Build history of the part. All positions in model axes, mm. A direction names the side the tool comes from. Give positions to 0.01 mm unless a question says otherwise; leave off trailing zeros. Loops run counter-clockwise (first coordinate to the right, second up) from the corner with the lowest first, then second, coordinate; pieces in that order, holes last. Notation, with made-up numbers: (66.25, 83) -> (73.25, 83) arc R11 ccw to (73.25, 97) -> close; hole circle Ø7 at (19, 59.25). An arc over 180 degrees is marked (long way). Answer as a JSON object with one key per item and string values. Group by question number.
Q1. Drop flat-ended pins along their axis: pin 1 (3 mm diameter, centred on x = 94, y = 0, fed in from +Z); pin 2 (12 mm diameter, centred on x = 1.5, y = 0, fed in from +Z). Give the stop position or say it passes through.
Q2. Two-plate mould, pull along Y, no slides. Class faces 3 (the flat face through (-100, 0, 3)), 4 (the flat face through (-1, 16, 13)), 5 (the flat face through (-1, -17.5, 9)), 6 (the flat face through (-1, 0, 5)): pulls with the +Y half, pulls with the -Y half, needs draft (parallel to the pull), parting line crosses it, or undercut.
Q3. Wall check: probe 1 along Y at (x, z) = (-2.5, 13.5); probe 2 along Y at (x, z) = (94, 3.45); probe 3 along Z at (x, y) = (32, 0.5). Give the ranges that are in metal, low to high. Write a range as from..to.
Q4. Band-saw the part on B-B, the plane z = 9. Write the cut outline in (x, y).
Q5. Tool access for faces 1 (the cylindrical face through (-96.5, 0.1, 2.5)), 2 (the flat face through (-1, 7, 13)): list every direction of +Z, -Z, +X, -X, +Y, -Y with a clear straight run to the whole face (end or side of a thin tool).
Q6. Band-saw the part on A-A, the plane y = 0. Write the cut outline in (x, z), plus the area to 3 significant figures.
from build123d import *

# Parameters (mm, degrees)
F0_W     = 200
F0_H     = 35
F1_DEPTH = 20
F2_R     = 2.5
F3_DEPTH = 25
F4_SIZE  = 1
F6_DEPTH = 240
F8_DEPTH = 250


with BuildPart() as f1:
    # F0 (on Top) → F1 (new body)
    with BuildSketch(Plane.XY):
        Rectangle(F0_W, F0_H)
    extrude(amount=F1_DEPTH)

    # F2 (on face) → F3 (cut)
    with BuildSketch(Plane.XY.offset(20)):
        with Locations((-94, 0)):
            Circle(F2_R)
        with Locations((94, 0)):
            Circle(F2_R)
    extrude(amount=-F3_DEPTH, mode=Mode.SUBTRACT)

    # F4
    f4_edges = [f1.edges().sort_by_distance(p)[0] for p in [
        (0, 17.5, 20),
        (100, 0, 20),
        (-100, 0, 20),
        (0, -17.5, 20),
        (-96.5, 0, 20),
        (91.5, 0, 20),
    ]]
    chamfer(f4_edges, length=F4_SIZE)

    # F5 (on face) → F6 (cut)
    with BuildSketch(Plane(origin=(-100, 0, 0), x_dir=(0, -1, 0), z_dir=(-1, 0, 0))):
        with BuildLine():
            Line((-13, 21.054447), (-16, 21.054447))
            Line((-16, 21.054447), (-16, 6.5))
            ThreePointArc((-16, 6.5), (-15.56066, 5.43934), (-14.5, 5))
            ThreePointArc((-14.5, 5), (-13.43934, 5.43934), (-13, 6.5))
            Line((-13, 6.5), (-13, 21.054447))
        make_face()
        with BuildLine():
            Line((-8.5, 21.054447), (-11.5, 21.054447))
            Line((-11.5, 21.054447), (-11.5, 6.5))
            ThreePointArc((-11.5, 6.5), (-11.06066, 5.43934), (-10, 5))
            ThreePointArc((-10, 5), (-8.93934, 5.43934), (-8.5, 6.5))
            Line((-8.5, 6.5), (-8.5, 21.054447))
        make_face()
        with BuildLine():
            Line((-4, 20.95042), (-7, 20.95042))
            Line((-7, 20.95042), (-7, 6.5))
            ThreePointArc((-7, 6.5), (-6.56066, 5.43934), (-5.5, 5))
            ThreePointArc((-5.5, 5), (-4.43934, 5.43934), (-4, 6.5))
            Line((-4, 6.5), (-4, 20.95042))
        make_face()
        with BuildLine():
            Line((11.5, 21.002434), (8.5, 21.002434))
            Line((8.5, 21.002434), (8.5, 6.5))
            ThreePointArc((8.5, 6.5), (8.93934, 5.43934), (10, 5))
            ThreePointArc((10, 5), (11.06066, 5.43934), (11.5, 6.5))
            Line((11.5, 6.5), (11.5, 21.002434))
        make_face()
        with BuildLine():
            Line((16, 21.002434), (13, 21.002434))
            Line((13, 21.002434), (13, 6.5))
            ThreePointArc((13, 6.5), (13.43934, 5.43934), (14.5, 5))
            ThreePointArc((14.5, 5), (15.56066, 5.43934), (16, 6.5))
            Line((16, 6.5), (16, 21.002434))
        make_face()
        with BuildLine():
            Line((7, 21.002434), (4, 21.002434))
            Line((4, 21.002434), (4, 6.5))
            ThreePointArc((4, 6.5), (4.43934, 5.43934), (5.5, 5))
            ThreePointArc((5.5, 5), (6.56066, 5.43934), (7, 6.5))
            Line((7, 6.5), (7, 21.002434))
        make_face()
    extrude(amount=-F6_DEPTH, mode=Mode.SUBTRACT)

    # F7 (on face) → F8 (cut)
    with BuildSketch(Plane(origin=(-100, 0, 0), x_dir=(0, -1, 0), z_dir=(-1, 0, 0))):
        with BuildLine():
            ThreePointArc((-4, 6.5), (-4.43934, 5.43934), (-5.5, 5))
            Line((-5.5, 5), (5.5, 5))
            ThreePointArc((5.5, 5), (4.43934, 5.43934), (4, 6.5))
            Line((4, 6.5), (4, 19))
            Line((4, 19), (-4, 19))
            Line((-4, 19), (-4, 6.5))
        make_face()
        with BuildLine():
            Line((5.5, 21.402081), (-5.5, 21.402081))
            Line((-5.5, 21.402081), (-5.5, 5))
            ThreePointArc((-5.5, 5), (-4.43934, 5.43934), (-4, 6.5))
            Line((-4, 6.5), (-4, 19))
            Line((-4, 19), (4, 19))
            Line((4, 19), (4, 6.5))
            ThreePointArc((4, 6.5), (4.43934, 5.43934), (5.5, 5))
            Line((5.5, 5), (5.5, 21.402081))
        make_face()
    extrude(amount=-F8_DEPTH, mode=Mode.SUBTRACT)


solid = f1.part
Worked answers:
{
 "1": {"pin 1": "through", "pin 2": "z = 5.09"},
 "2": {"face 3": "needs draft", "face 4": "undercut", "face 5": "pulls with the -Y half", "face 6": "undercut"},
 "3": {"probe 1": "-17.5..-16, -13..-11.5, -8.5..-7, 7..8.5, 11.5..13, 16..17.5", "probe 2": "-17.5..-2.5, 2.5..17.5", "probe 3": "0..5"},
 "4": {"outline": "(-100, -17.5) -> (100, -17.5) -> (100, -16) -> (-100, -16) -> close; (-100, -13) -> (100, -13) -> (100, -11.5) -> (-100, -11.5) -> close; (-100, -8.5) -> (100, -8.5) -> (100, -7) -> (-100, -7) -> close; (-100, 7) -> (100, 7) -> (100, 8.5) -> (-100, 8.5) -> close; (-100, 11.5) -> (100, 11.5) -> (100, 13) -> (-100, 13) -> close; (-100, 16) -> (100, 16) -> (100, 17.5) -> (-100, 17.5) -> close"},
 "5": {"face 1": "+Z, -Z", "face 2": "+Z, +X, -X"},
 "6": {"outline": "(-100, 0) -> (-96.5, 0) -> (-96.5, 5) -> (-100, 5) -> close; (-91.5, 0) -> (91.5, 0) -> (91.5, 5) -> (-91.5, 5) -> close; (96.5, 0) -> (100, 0) -> (100, 5) -> (96.5, 5) -> close", "area": "950 mm2"}
}
